from build123d import *

# Parameters (mm, degrees)
SKETCH4_W                      = 111.737645783
SKETCH4_H                      = 62.825705526
BOSS_EXTRUDE3_DEPTH            = 20.22630919
SKETCH5_W                      = 103.737645783
SKETCH5_H                      = 6.825139403
CUT_EXTRUDE1_DEPTH             = 131.749158903
CUT_EXTRUDE2_DEPTH             = 131.749158903
SKETCH7_W                      = 87.737645783
SKETCH7_H                      = 14
CUT_EXTRUDE3_DEPTH             = 1
SKETCH8_W                      = 87.737645783
SKETCH8_H                      = 14
CUT_EXTRUDE4_DEPTH             = 1
DRAFT1_ANGLE                   = 17.058179216
F_16_0_16_DIAMETER_HOLE1_D     = 16
F_16_0_16_DIAMETER_HOLE1_DEPTH = 4
F_16_0_16_DIAMETER_HOLE2_D     = 16
F_16_0_16_DIAMETER_HOLE2_DEPTH = 4
F_4_0_4_DIAMETER_HOLE1_D       = 4
F_4_0_4_DIAMETER_HOLE1_DEPTH   = 6
F_4_0_4_DIAMETER_HOLE2_D       = 4
F_4_0_4_DIAMETER_HOLE2_DEPTH   = 68.031973705
M10_CLEARANCE_HOLE1_D          = 11.9
CHAMFER1_SIZE                  = 6.825139403
CHAMFER1_SIZE2                 = 2.933140798
CHAMFER2_SIZE                  = 6.825139403
CHAMFER2_SIZE2                 = 2.933140798
SKETCH19_W                     = 111.737645783
SKETCH19_H                     = 56.000566123
BOSS_EXTRUDE4_DEPTH            = 2
FILLET7_R                      = 4
CHAMFER3_SIZE                  = 11
CHAMFER4_SIZE                  = 11
FILLET9_R                      = 24
FILLET10_R                     = 24
CUT_EXTRUDE6_DEPTH             = 1
FILLET13_R                     = 4
FILLET14_R                     = 4
FILLET15_R                     = 4


# Some blends are built 0.0001 mm under size
with BuildPart() as part:
    # Sketch4 → Boss-Extrude3 (new body)
    with BuildSketch(Plane(origin=(0, 0, 67.988216463), x_dir=(-1, 0, 0), z_dir=(0, 0, -1))):
        with Locations((-27.467757585, 67.284935079)):
            Rectangle(SKETCH4_W, SKETCH4_H)
    extrude(amount=-BOSS_EXTRUDE3_DEPTH)

    # Sketch5 → Cut-Extrude1 (cut, through all)
    with BuildSketch(Plane.XY.offset(88.214525653)):
        with Locations((27.467757585, 95.285218141)):
            Rectangle(SKETCH5_W, SKETCH5_H)
    extrude(amount=-CUT_EXTRUDE1_DEPTH, mode=Mode.SUBTRACT)

    # Sketch6 → Cut-Extrude2 (cut, through all)
    with BuildSketch(Plane.XY.offset(88.214525653)):
        with BuildLine():
            Line((-21.401065306, 66.205832154), (-21.401065306, 42.872082316))
            Line((-21.401065306, 42.872082316), (76.336580477, 42.872082316))
            Line((76.336580477, 42.872082316), (76.336580477, 66.098543331))
            ThreePointArc((76.336580477, 66.098543331), (63.931745492, 73.877367201), (76.336580477, 81.65619107))
            Line((76.336580477, 81.65619107), (76.336580477, 84.872648439))
            Line((76.336580477, 84.872648439), (-21.401065306, 84.872648439))
            Line((-21.401065306, 84.872648439), (-21.401065306, 81.548902247))
            ThreePointArc((-21.401065306, 81.548902247), (-8.768867408, 73.877367201), (-21.401065306, 66.205832154))
        make_face()
    extrude(amount=-CUT_EXTRUDE2_DEPTH, mode=Mode.SUBTRACT)

    # Sketch7 → Cut-Extrude3 (cut)
    with BuildSketch(Plane(origin=(0, 91.872648439, 0), x_dir=(-1, 0, 0), z_dir=(0, 1, 0))):
        with Locations((-27.467757585, 74.988216463)):
            Rectangle(SKETCH7_W, SKETCH7_H)
    extrude(amount=-CUT_EXTRUDE3_DEPTH, mode=Mode.SUBTRACT)

    # Sketch8 → Cut-Extrude4 (cut)
    with BuildSketch(Plane.XZ.offset(-35.872082316)):
        with Locations((27.467757585, 74.988216463)):
            Rectangle(SKETCH8_W, SKETCH8_H)
    extrude(amount=-CUT_EXTRUDE4_DEPTH, mode=Mode.SUBTRACT)

    # Draft1
    draft1_faces = [part.faces().sort_by_distance(p)[0] for p in [
        (-26.401065306, 98.697787842, 78.101371058),
        (81.336580477, 98.697787842, 78.101371058),
    ]]
    draft(draft1_faces, Plane.XY.offset(88.214525653), DRAFT1_ANGLE)

    # Ø16.0 (16) Diameter Hole1
    with Locations(Plane.ZY.offset(28.401065306)):
        with Locations((77.644129293, 88.158482369)):
            Hole(F_16_0_16_DIAMETER_HOLE1_D / 2, depth=F_16_0_16_DIAMETER_HOLE1_DEPTH)

    # Ø16.0 (16) Diameter Hole2
    with Locations(Plane(origin=(83.336580477, 0, 0), x_dir=(0, 0, -1), z_dir=(1, 0, 0))):
        with Locations((-77.930295014, 87.866076089)):
            Hole(F_16_0_16_DIAMETER_HOLE2_D / 2, depth=F_16_0_16_DIAMETER_HOLE2_DEPTH)

    # Ø4.0 (4) Diameter Hole1
    with Locations(Plane(origin=(0, 90.872648439, 0), x_dir=(1, 0, 0), z_dir=(0, 1, 0))):
        with Locations((40.713339239, -75.969517026), (28.761431707, -75.969517026), (16.662423773, -75.969517026)):
            Hole(F_4_0_4_DIAMETER_HOLE1_D / 2, depth=F_4_0_4_DIAMETER_HOLE1_DEPTH)

    # Ø4.0 (4) Diameter Hole2
    with Locations(Plane(origin=(0, 36.872082316, 0), x_dir=(-1, 0, 0), z_dir=(0, -1, 0))):
        with Locations((-40.713339239, -75.969517026), (-28.761431707, -75.969517026), (-16.662423773, -75.969517026)):
            Hole(F_4_0_4_DIAMETER_HOLE2_D / 2, depth=F_4_0_4_DIAMETER_HOLE2_DEPTH)

    # M10 Clearance Hole1 (through all)
    with Locations(Plane(origin=(0, 0, 67.988216463), x_dir=(-1, 0, 0), z_dir=(0, 0, -1))):
        with Locations((-72.573135404, 73.877367201), (17.414428357, 73.877367201)):
            Hole(M10_CLEARANCE_HOLE1_D / 2)

    # Chamfer1
    chamfer1_edges = [part.edges().sort_by_distance(p)[0] for p in [
        (81.336580477, 98.697787842, 88.214525653),
    ]]
    chamfer1_side = [part.faces().sort_by_distance(p)[0] for p in [
        (27.467757585, 37.153970406, 88.214525653),
    ]]
    chamfer(chamfer1_edges, length=CHAMFER1_SIZE, length2=CHAMFER1_SIZE2, reference=chamfer1_side[0])

    # Chamfer2
    chamfer2_edges = [part.edges().sort_by_distance(p)[0] for p in [
        (-26.401065306, 98.697787842, 88.214525653),
    ]]
    chamfer2_side = [part.faces().sort_by_distance(p)[0] for p in [
        (82.054692387, 63.872365377, 88.214525653),
    ]]
    chamfer(chamfer2_edges, length=CHAMFER2_SIZE, length2=CHAMFER2_SIZE2, reference=chamfer2_side[0])

    # Sketch19 → Boss-Extrude4 (add)
    with BuildSketch(Plane.XY.offset(88.214525653)):
        with Locations((27.467757585, 63.872365378)):
            Rectangle(SKETCH19_W, SKETCH19_H)
    extrude(amount=BOSS_EXTRUDE4_DEPTH)

    # Fillet7
    # the kernel refuses this fillet: 4 mm, written as the material it takes off along each edge
    with BuildSketch(Plane(origin=(93.336580477, 91.872648439, 90.214525653), x_dir=(0, 0, -1), z_dir=(-1, 0, 0))) as fillet7_piece_1_section:
        with BuildLine():
            CenterArc((FILLET7_R, FILLET7_R), FILLET7_R, 180, 90)
            Line((0, FILLET7_R), (0, 0))
            Line((0, 0), (FILLET7_R, 0))
        make_face()
    fillet7_piece_1 = extrude(amount=131.737645784, mode=Mode.PRIVATE)
    fillet7_piece_1 = split(fillet7_piece_1, bisect_by=Plane(origin=(81.336580477, 90.577181296, 88.687181842), z_dir=(0, 0.34275303765814863, 0.9394255453074032)), keep=Keep.TOP, mode=Mode.PRIVATE)
    add(fillet7_piece_1, mode=Mode.SUBTRACT)
    with BuildSketch(Plane(origin=(93.336580477, 91.872648439, 90.214525653), x_dir=(0, 0, -1), z_dir=(-1, 0, 0))) as fillet7_piece_2_section:
        with BuildLine():
            CenterArc((FILLET7_R, FILLET7_R), FILLET7_R, 180, 90)
            Line((0, FILLET7_R), (0, 0))
            Line((0, 0), (FILLET7_R, 0))
        make_face()
    fillet7_piece_2 = extrude(amount=131.737645784, mode=Mode.PRIVATE)
    fillet7_piece_2 = split(fillet7_piece_2, bisect_by=Plane(origin=(-24.401065306, 91.673256094, 87.815354023), z_dir=(1, 0, 0)), keep=Keep.TOP, mode=Mode.PRIVATE)
    fillet7_piece_2 = split(fillet7_piece_2, bisect_by=Plane(origin=(79.336580477, 91.673256094, 87.815354023), z_dir=(-1, 0, 0)), keep=Keep.TOP, mode=Mode.PRIVATE)
    add(fillet7_piece_2, mode=Mode.SUBTRACT)

    # Chamfer3
    chamfer3_edges = [part.edges().sort_by_distance(p)[0] for p in [
        (83.336580477, 35.872082316, 79.101371058),
    ]]
    chamfer(chamfer3_edges, length=CHAMFER3_SIZE)

    # Chamfer4
    chamfer4_edges = [part.edges().sort_by_distance(p)[0] for p in [
        (-28.401065306, 35.872082316, 79.101371058),
    ]]
    chamfer(chamfer4_edges, length=CHAMFER4_SIZE)

    # Fillet9
    fillet9_edges = [part.edges().sort_by_distance(p)[0] for p in [
        (83.336580477, 46.872082316, 79.101371058),
    ]]
    fillet(fillet9_edges, radius=FILLET9_R)

    # Fillet10
    fillet10_edges = [part.edges().sort_by_distance(p)[0] for p in [
        (-28.401065306, 46.872082316, 79.101371058),
    ]]
    fillet(fillet10_edges, radius=FILLET10_R)

    # Sketch21 → Cut-Extrude6 (cut)
    with BuildSketch(Plane.XY.offset(90.214525653)):
        Polygon((-26.391485045, 85.865514682), (-26.391485045, 66.022635818), (27.807921223, 54.570460017), (81.893939612, 68.063617644), (81.893939612, 85.865514682), align=None)
    extrude(amount=-CUT_EXTRUDE6_DEPTH, mode=Mode.SUBTRACT)

    # Fillet13
    fillet13_edges = [part.edges().sort_by_distance(p)[0] for p in [
        (-28.401065306, 102.231129511, 76.699318929),
    ]]
    fillet(fillet13_edges, radius=FILLET13_R - 0.0001)  # a hair under: the kernel refuses the full size

    # Fillet14
    fillet14_edges = [part.edges().sort_by_distance(p)[0] for p in [
        (83.336580477, 102.231129511, 76.699318929),
    ]]
    fillet(fillet14_edges, radius=FILLET14_R - 0.0001)  # a hair under: the kernel refuses the full size

    # Fillet15
    fillet15_edges = [part.edges().sort_by_distance(p)[0] for p in [
        (27.467757585, 35.872082316, 90.214525653),
    ]]
    fillet(fillet15_edges, radius=FILLET15_R)


solid = part.part
Build history of the part. All positions in model axes, mm. A direction names the side the tool comes from. Coordinates: 2 decimals unless noted, no trailing zeros. Order: outer loops, then holes, each group sorted by start corner. A loop starts at its lowest first (then second) coordinate and runs counter-clockwise, first axis right, second up. Notation, with made-up numbers: (-13, -10) -> (32, -10) arc R15 cw to (32, -2) -> close; hole circle Ø11 at (55, 53.25). An arc over 180 degrees is marked (long way). One line per item, written item: value.
(1) Slice it at A-A, the plane x = 16.5. List the corners of the cut face in (y, z).
Checked values:
outline: (35.87, 81.99) -> (36.87, 81.99) -> (36.87, 77.96) -> (42.87, 77.96) -> (42.87, 88.21) -> (84.87, 88.21) -> (84.87, 77.96) -> (90.87, 77.96) -> (90.87, 81.99) -> (91.87, 81.99) -> (91.87, 86.21) arc R4 ccw to (87.87, 90.21) -> (85.87, 90.21) -> (85.87, 89.21) -> (56.96, 89.21) -> (56.96, 90.21) -> (39.87, 90.21) arc R4 ccw to (35.87, 86.21) -> close; (36.87, 67.99) -> (42.87, 67.99) -> (42.87, 73.98) -> (36.87, 73.98) -> close; (84.87, 67.99) -> (90.87, 67.99) -> (90.87, 73.98) -> (84.87, 73.98) -> close
(2) Tool access for faces 5 (the flat face through (-17, 74, 88.215)), 6 (the flat face through (27, 74, 89.215)), 7 (the flat face through (27, 36.872, 74)), 8 (the flat face through (79.337, 87, 78)): list every direction of +Z, -Z, +X, -X, +Y, -Y with a clear straight run to the whole face (end or side of a thin tool).
Checked values:
face 5: -Z
face 6: +Z
face 7: -Z, -Y
face 8: +X
(3) Slice it at D-D, the plane y = 62.5. List the corners of the cut face in (x, z), plus the area to 3 significant figures.
Checked values:
outline: (-28.4, 67.99) -> (-21.4, 67.99) -> (-21.4, 88.21) -> (76.34, 88.21) -> (76.34, 67.99) -> (83.34, 67.99) -> (83.34, 90.21) -> (59.59, 90.21) -> (59.59, 89.21) -> (-9.72, 89.21) -> (-9.72, 90.21) -> (-28.4, 90.21) -> close
area: 437 mm2
(4) Probe line 1 (Y direction, x = 59.5, z = 79.5); line 2 (X direction, y = 84, z = 80.5); line 3 (X direction, y = 89, z = 77.5). List the from-to ranges inside material, lowest first. Write a range as [from, to].
Checked values:
line 1: [36.87, 42.87], [84.87, 90.87]
line 2: [-24.4, -21.4], [76.34, 79.34]
line 3: [-24.4, 15.37], [17.95, 27.47], [30.05, 39.43], [42, 79.34]
(5) Slice it at B-B, the plane x = 3. List the corners of the cut face in (y, z), plus the area to 3 significant figures.
Checked values:
outline: (35.87, 81.99) -> (36.87, 81.99) -> (36.87, 67.99) -> (42.87, 67.99) -> (42.87, 88.21) -> (84.87, 88.21) -> (84.87, 67.99) -> (90.87, 67.99) -> (90.87, 81.99) -> (91.87, 81.99) -> (91.87, 86.21) arc R4 ccw to (87.87, 90.21) -> (85.87, 90.21) -> (85.87, 89.21) -> (59.81, 89.21) -> (59.81, 90.21) -> (39.87, 90.21) arc R4 ccw to (35.87, 86.21) -> close
area: 334 mm2
(6) Drop flat-ended pins along their axis: pin 1 Ø12 at (x, z) = (26, 84) entering from +Y; pin 2 Ø2.5 at (x, z) = (40.71, 75.97) entering from -Y; pin 3 Ø4 at (x, y) = (4, 62) entering from -Z; pin 4 Ø0.5 at (x, z) = (32.5, 89.5) entering from -Y. Give the stop position or say it passes through.
Checked values:
pin 1: y = 91.87
pin 2: through
pin 3: z = 88.21
pin 4: y = 37.27
(7) Mould opens along Z. For faces 1 (the cylindrical face through (40.974, 87.831, 73.987)), 2 (the flat face through (27, 64, 88.215)), 3 (the cylindrical face through (16.402, 39.914, 73.987)), 4 (the cylindrical face through (71.28, 68.07, 78.24)) say: pulls with the +Z half, pulls with the -Z half, needs draft (parallel to the pull), parting line crosses it, or undercut.
Checked values:
face 1: undercut
face 2: pulls with the -Z half
face 3: undercut
face 4: needs draft
(8) Slice it at C-C, the plane z = 72.75. Count the separate pieces of the cut face and the enclosed holes in it, plus the area to 3 significant figures.
Checked values:
separate pieces: 3
enclosed holes: 3
area: 1,960 mm2
